```python
from build123d import *

# Parameters (mm, degrees)
F0_R     = 6
F1_DEPTH = 12
F2_R     = 6
F3_DEPTH = 6
F5_D     = 9
F6_SIZE  = 0.5


with BuildPart() as f1:
    # F0 (on Front) → F1 (new body, symmetric)
    with BuildSketch(Plane.XZ):
        Polygon((18, 18), (0, 18), (-18, 18), (-18, -1), (-35, -1), (-35, -25), (0, -25), (35, -25), (35, -1), (18, -1), align=None)
        Circle(F0_R, mode=Mode.SUBTRACT)
    extrude(amount=F1_DEPTH, both=True)

    # F2 (on face) → F3 (join)
    with BuildSketch(Plane.XZ.offset(12)):
        Polygon((18, 18), (-18, 18), (-18, -1), (-18, -18), (18, -18), (18, -1), align=None)
        Circle(F2_R, mode=Mode.SUBTRACT)
    extrude(amount=F3_DEPTH)

    # F5 (through all)
    with Locations(Plane(origin=(0, 0, -25), x_dir=(1, 0, 0), z_dir=(0, 0, -1))):
        with Locations((-26, 0), (26, 0)):
            Hole(F5_D / 2)

    # F6
    f6_edges = [f1.edges().sort_by_distance(p)[0] for p in [
        (18, -3, 18),
        (-18, -3, 18),
        (0, -18, 18),
        (-18, -18, 0),
        (0, -18, -18),
        (18, -18, 0),
        (-6, -18, 0),
        (35, 0, -25),
        (35, 12, -13),
        (35, 0, -1),
        (35, -12, -13),
        (26.5, 12, -1),
        (18, 12, 8.5),
        (0, 12, 18),
        (-26.5, 12, -1),
        (-18, 12, 8.5),
        (-18, 0, -1),
        (-18, -12, -9.5),
        (-18, -15, -18),
        (18, -15, -18),
        (18, -12, -9.5),
        (18, 0, -1),
        (0, 12, -25),
        (-35, 0, -1),
        (-35, 12, -13),
        (-35, 0, -25),
        (-35, -12, -13),
        (0, -12, -25),
        (0, -12, -18),
    ]]
    chamfer(f6_edges, length=F6_SIZE)


solid = f1.part
```
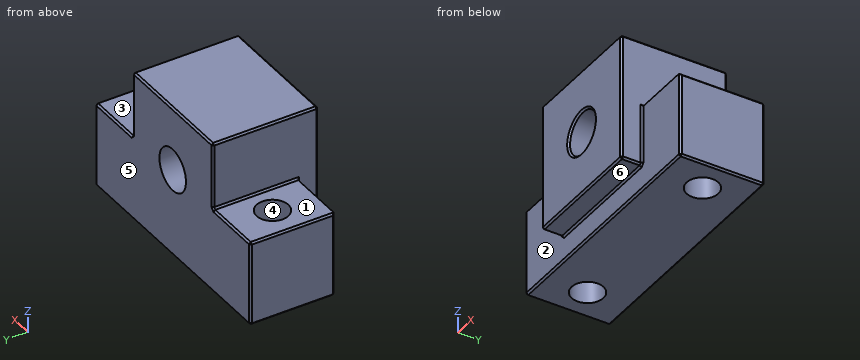
Input: part model. Units: mm. Frame: model coordinates. Face numbers are marked on the shaded views. A direction names the side the tool comes from. Coordinates: 2 decimals unless noted, no trailing zeros. Loops run counter-clockwise (first coordinate to the right, second up) from the corner with the lowest first, then second, coordinate; pieces in that order, holes last. Notation, with made-up numbers: (-32, 75.5) -> (-5, 75.5) arc R22 cw to (-5, 91.5) -> close; hole circle Ø5 at (-18.5, 15). An arc over 180 degrees is marked (long way). Use a Markdown table: item, result.
1) Material intervals for line 1 along Z through (x, y) = (0, 1.75); line 2 along X through (y, z) = (-14.25, -7); line 3 along Y through (x, z) = (-26, -13), sorted ascending. Write a range as from..to.
Results found:
| item | result |
|---|---|
| line 1 | z = -25..-6, 6..18 |
| line 2 | x = -18..18 |
| line 3 | y = -12..-4.5, 4.5..12 |
2) Pull-direction query (Y, two-part tool) for the marked faces 4, 5 and 6; classes: released by +Y, released by -Y, zero draft, split by the parting line, or undercut.
Results found:
| item | result |
|---|---|
| face 4 | undercut |
| face 5 | released by +Y |
| face 6 | zero draft |
3) Cut plane B-B (x = 0). Return the cut outline in (y, z).
Results found:
| item | result |
|---|---|
| outline | (-18, -17.5) -> (-17.5, -18) -> (-12.5, -18) -> (-12, -18.5) -> (-12, -24.5) -> (-11.5, -25) -> (11.5, -25) -> (12, -24.5) -> (12, -6) -> (-17.5, -6) -> (-18, -6.5) -> close; (-18, 6.5) -> (-17.5, 6) -> (12, 6) -> (12, 17.5) -> (11.5, 18) -> (-17.5, 18) -> (-18, 17.5) -> close |
4) Cut plane A-A (y = 0). Return the cut outline in (x, z).
Results found:
| item | result |
|---|---|
| outline | (-35, -24.5) -> (-34.5, -25) -> (-30.5, -25) -> (-30.5, -1) -> (-34.5, -1) -> (-35, -1.5) -> close; (-21.5, -25) -> (21.5, -25) -> (21.5, -1) -> (18.5, -1) -> (18, -0.5) -> (18, 17.5) -> (17.5, 18) -> (-17.5, 18) -> (-18, 17.5) -> (-18, -0.5) -> (-18.5, -1) -> (-21.5, -1) -> close; (30.5, -25) -> (34.5, -25) -> (35, -24.5) -> (35, -1.5) -> (34.5, -1) -> (30.5, -1) -> close; hole circle Ø12 at (0, 0) |
5) Cut plane D-D (z = 11). Return the cut outline in (x, y), then the cut area to 3 significant figures.
Results found:
| item | result |
|---|---|
| outline | (-18, -17.5) -> (-17.5, -18) -> (17.5, -18) -> (18, -17.5) -> (18, 11.5) -> (17.5, 12) -> (-17.5, 12) -> (-18, 11.5) -> close |
| area | 1,080 mm2 |
6) Access query for the marked faces 1, 2 and 3. Directions: +Z, -Z, +X, -X, +Y, -Y. A direction counts if a zero-diameter tool reaches every point of the face in a straight line with its end or side. Return the directions, or none.
Results found:
| item | result |
|---|---|
| face 1 | +Z, -X, +Y, -Y |
| face 2 | -Z, -Y |
| face 3 | +Z, +X, +Y, -Y |
7) Contact query for flat-ended pins moving along their axis: pin 1 (5 mm diameter, centred on x = 27.5, y = 3.5, fed in from +Z); pin 2 (5.5 mm diameter, centred on x = 5.5, y = -14.5, fed in from -Z). Output: stop coordinate, or through.
Results found:
| item | result |
|---|---|
| pin 1 | stops at z = -1 |
| pin 2 | stops at z = -24.75 |
8) Cut plane C-C (y = 8). Return the cut outline in (x, z), then the cut area to 3 significant figures.
Results found:
| item | result |
|---|---|
| outline | (-35, -24.5) -> (-34.5, -25) -> (34.5, -25) -> (35, -24.5) -> (35, -1.5) -> (34.5, -1) -> (18.5, -1) -> (18, -0.5) -> (18, 17.5) -> (17.5, 18) -> (-17.5, 18) -> (-18, 17.5) -> (-18, -0.5) -> (-18.5, -1) -> (-34.5, -1) -> (-35, -1.5) -> close; hole circle Ø12 at (0, 0) |
| area | 2,250 mm2 |
